CAD build for the part. Positions are in the model's coordinates, mm. A direction names the side the tool comes from. Give positions to 0.01 mm unless a question says otherwise; leave off trailing zeros. Write each loop counter-clockwise with the first axis right and the second up, starting at its lowest first coordinate (ties: lowest second). Pieces come first, ordered by that corner, then holes. Notation, with made-up numbers: M -14,52 L 40,52 A9 ccw 40,69 Z; hole C -25.75,-40 d2. An arc over 180 degrees is marked long. One line per question, with ' | ' between items. Start each with the question number.
1. Flat gauge pins, fed straight in: pin 1 (3 mm diameter, centred on x = -50, z = 0, fed in from -Y); pin 2 (1 mm diameter, centred on x = -61, y = 0.5, fed in from +Z); pin 3 (1 mm diameter, centred on x = -93, y = 0.5, fed in from +Z). Where does each tip first touch, or does it go through?
2. Cut at D-D, the plane z = 75.5. Write the cut outline in (x, y).
3. Cut at B-B, the plane x = 4. Write the cut outline in (y, z), then the cut area to 3 significant figures.
4. Pull direction X, two halves, no side cores. Call faces 1 (the face through (46.4, 2, -7.1)), 2 (the face through (72, 1, 89)), 3 (the face through (123, 1, -89)), 4 (the face through (-75, 1, -20)): released by +X, released by -X, zero draft, split by the parting line, or undercut.
5. Cut at A-A, the plane z = -38. Write the cut outline in (x, y), then the cut area to 3 significant figures.
6. Wall check: L1, parallel to Z at x = 30, y = 1.6; L2, parallel to X at y = 1.85, z = -2.5; L3, parallel to X at y = 1.35, z = -69. Give the ranges that are in metal, low to high.
7. Which spindle directions (+Z, -Z, +X, -X, +Y, -Y) get a long thin tool onto all of the face, cutting with end or side? Do faces 5 (the face through (-75, 1, 20)), 6 (the face through (15, 1, -20)), 7 (the face through (21, 1, 48)). Say none if no direction does.
8. Cut at C-C, the plane y = 1.5. Count the separate pieces of the cut face and the enclosed holes in it, then the cut area to 3 significant figures.
```python
from build123d import *

# Parameters (mm, degrees)
SKETCH1_R           = 1.75
SKETCH1_R_2         = 2
SKETCH1_R_3         = 1.25
SKETCH1_W           = 2.8
SKETCH1_H           = 29
BOSS_EXTRUDE1_DEPTH = 2
SKETCH3_R           = 1.75
SKETCH3_W           = 17
SKETCH3_H           = 37.6
SKETCH3_W_2         = 2
SKETCH3_H_2         = 50
SKETCH3_W_3         = 50
SKETCH3_H_3         = 40
SKETCH3_W_4         = 10
SKETCH3_H_4         = 28.52743249
CUT_EXTRUDE1_DEPTH  = 10
FILLET1_R           = 2
FILLET2_R           = 5
FILLET3_R           = 10
CUT_EXTRUDE2_DEPTH  = 10
SKETCH5_R           = 1.75
SKETCH5_R_2         = 1.5
CUT_EXTRUDE3_DEPTH  = 10
FILLET4_R           = 5


with BuildPart() as part:
    # Sketch1 → Boss-Extrude1 (new body)
    with BuildSketch(Plane(origin=(0, 0, 0), x_dir=(1, 0, 0), z_dir=(0, 1, 0))):
        Polygon((20, 90), (125, 90), (125, -90), (20, -90), (20, -25), (-100, -25), (-100, 25), (20, 25), align=None)
        with Locations((120, -85)):
            Circle(SKETCH1_R, mode=Mode.SUBTRACT)
        with Locations((120, 85)):
            Circle(SKETCH1_R, mode=Mode.SUBTRACT)
        with Locations((75, -67)):
            Circle(SKETCH1_R, mode=Mode.SUBTRACT)
        with Locations((120, -30)):
            Circle(SKETCH1_R, mode=Mode.SUBTRACT)
        with Locations((75, -30)):
            Circle(SKETCH1_R, mode=Mode.SUBTRACT)
        with Locations((75, 67)):
            Circle(SKETCH1_R, mode=Mode.SUBTRACT)
        with Locations((-95, -18.5)):
            Circle(SKETCH1_R_2, mode=Mode.SUBTRACT)
        with Locations((-95, 18.5)):
            Circle(SKETCH1_R_2, mode=Mode.SUBTRACT)
        with Locations((-81, 8)):
            Circle(SKETCH1_R_3, mode=Mode.SUBTRACT)
        with Locations((-81, -8)):
            Circle(SKETCH1_R_3, mode=Mode.SUBTRACT)
        with Locations((120, 30)):
            Circle(SKETCH1_R, mode=Mode.SUBTRACT)
        with Locations((75, 30)):
            Circle(SKETCH1_R, mode=Mode.SUBTRACT)
        with Locations((30, -43)):
            Circle(SKETCH1_R, mode=Mode.SUBTRACT)
        with Locations((30, 43)):
            Circle(SKETCH1_R, mode=Mode.SUBTRACT)
        with Locations((-93, 0)):
            Rectangle(SKETCH1_W, SKETCH1_H, mode=Mode.SUBTRACT)
    extrude(amount=BOSS_EXTRUDE1_DEPTH)

    # Sketch3 → Cut-Extrude1 (cut)
    with BuildSketch(Plane(origin=(0, 2, 0), x_dir=(1, 0, 0), z_dir=(0, 1, 0))):
        with Locations((77.5, 57)):
            Circle(SKETCH3_R)
        with Locations((117.5, 57)):
            Circle(SKETCH3_R)
        with Locations((117.5, -57)):
            Circle(SKETCH3_R)
        with Locations((77.5, -57)):
            Circle(SKETCH3_R)
        with Locations((81.63, 18.69)):
            Circle(SKETCH3_R)
        with Locations((118.37, 18.69)):
            Circle(SKETCH3_R)
        with Locations((81.63, -18.69)):
            Circle(SKETCH3_R)
        with Locations((118.37, -18.69)):
            Circle(SKETCH3_R)
        with Locations((33, 0)):
            Circle(SKETCH3_R)
        with Locations((97.5, 52.2)):
            Rectangle(SKETCH3_W, SKETCH3_H)
        with Locations((97.5, -52.2)):
            Rectangle(SKETCH3_W, SKETCH3_H)
        Polygon((85.980499335, 14.263716245), (85.980499335, 21.263716245), (114.019500665, 21.263716245), (114.019500665, 14.263716245), (115.019500665, 14.263716245), (115.019500665, -14.263716245), (114.019500665, -14.263716245), (114.019500665, -21.263716245), (85.980499335, -21.263716245), (85.980499335, -14.263716245), (78.980499335, -14.263716245), (78.980499335, 14.263716245), align=None)
        with Locations((45, 0)):
            Rectangle(SKETCH3_W_2, SKETCH3_H_2)
        with Locations((45, -70)):
            Rectangle(SKETCH3_W_3, SKETCH3_H_3)
        with Locations((45, 70)):
            Rectangle(SKETCH3_W_3, SKETCH3_H_3)
        with Locations((68.980499335, 0)):
            Rectangle(SKETCH3_W_4, SKETCH3_H_4)
    extrude(amount=-CUT_EXTRUDE1_DEPTH, mode=Mode.SUBTRACT)

    # Fillet1
    fillet1_edges = [part.edges().sort_by_distance(p)[0] for p in [
        (-100, 1, 25),
        (-100, 1, -25),
    ]]
    fillet(fillet1_edges, radius=FILLET1_R)

    # Fillet2
    fillet2_edges = [part.edges().sort_by_distance(p)[0] for p in [
        (20, 1, -50),
        (125, 1, 90),
        (125, 1, -90),
        (20, 1, 50),
        (70, 1, -90),
        (70, 1, 90),
    ]]
    fillet(fillet2_edges, radius=FILLET2_R)

    # Fillet3
    fillet3_edges = [part.edges().sort_by_distance(p)[0] for p in [
        (70, 1, 50),
        (70, 1, -50),
    ]]
    fillet(fillet3_edges, radius=FILLET3_R)

    # Sketch4 → Cut-Extrude2 (cut)
    with BuildSketch(Plane(origin=(0, 2, 0), x_dir=(1, 0, 0), z_dir=(0, 1, 0))):
        with BuildLine():
            ThreePointArc((118.37, 18.69), (121.357436867, 17.452563133), (120.12, 20.44))
            ThreePointArc((120.12, 20.44), (117.132563133, 21.677436867), (118.37, 18.69))
        make_face()
        with BuildLine():
            ThreePointArc((120.12, -20.44), (121.357436867, -17.452563133), (118.37, -18.69))
            ThreePointArc((118.37, -18.69), (117.132563133, -21.677436867), (120.12, -20.44))
        make_face()
        with BuildLine():
            ThreePointArc((79.88, -20.44), (82.867436867, -21.677436867), (81.63, -18.69))
            ThreePointArc((81.63, -18.69), (78.642563133, -17.452563133), (79.88, -20.44))
        make_face()
        with BuildLine():
            ThreePointArc((79.88, 20.44), (78.642563133, 17.452563133), (81.63, 18.69))
            ThreePointArc((81.63, 18.69), (82.867436867, 21.677436867), (79.88, 20.44))
        make_face()
    extrude(amount=-CUT_EXTRUDE2_DEPTH, mode=Mode.SUBTRACT)

    # Sketch5 → Cut-Extrude3 (cut)
    with BuildSketch(Plane(origin=(0, 2, 0), x_dir=(1, 0, 0), z_dir=(0, 1, 0))):
        with Locations((-70, 0)):
            Circle(SKETCH5_R)
        with Locations((-50, 0)):
            Circle(SKETCH5_R)
        with Locations((-30, 0)):
            Circle(SKETCH5_R)
        with Locations((-10, 0)):
            Circle(SKETCH5_R)
        with Locations((10, 0)):
            Circle(SKETCH5_R)
        with Locations((58.980499335, 10)):
            Circle(SKETCH5_R_2)
        with Locations((58.980499335, -10)):
            Circle(SKETCH5_R_2)
        with Locations((-21.019500665, 10)):
            Circle(SKETCH5_R_2)
        with Locations((-21.019500665, -10)):
            Circle(SKETCH5_R_2)
        Polygon((20, 25), (-80, 25), (-70, 15), (10, 15), align=None)
        Polygon((-70, -15), (10, -15), (20, -25), (-80, -25), align=None)
    extrude(amount=-CUT_EXTRUDE3_DEPTH, mode=Mode.SUBTRACT)

    # Fillet4
    fillet4_edges = [part.edges().sort_by_distance(p)[0] for p in [
        (-80, 1, -25),
        (-70, 1, -15),
        (-70, 1, 15),
        (-80, 1, 25),
    ]]
    fillet(fillet4_edges, radius=FILLET4_R)


solid = part.part
```
Here are the results:
1) pin 1: through | pin 2: z = 15 | pin 3: z = 25
2) outline: M 70,0 L 125,0 L 125,2 L 70,2 Z
3) outline: M 0,-15 L 2,-15 L 2,15 L 0,15 Z | area: 60.0 mm^2
4) face 1: zero draft | face 2: released by -X | face 3: released by +X | face 4: undercut
5) outline: M 20,0 L 89,0 L 89,2 L 20,2 Z; M 106,0 L 125,0 L 125,2 L 106,2 Z | area: 176 mm^2
6) L1: -50 to -44.75, -41.25 to 41.25, 44.75 to 50 | L2: -100 to -94.4, -91.6 to 44, 46 to 63.98, 73.98 to 78.98, 115.02 to 125 | L3: 70 to 89, 106 to 125
7) face 5: +Z, +Y, -Y | face 6: -Z, +Y, -Y | face 7: +Z, -X, +Y, -Y
8) separate pieces: 1 | enclosed holes: 38 | area: 15,600 mm^2
